CAD build for the part. Positions are in the model's coordinates, mm. Give positions to 0.01 mm unless a question says otherwise; leave off trailing zeros. Write each loop counter-clockwise with the first axis right and the second up, starting at its lowest first coordinate (ties: lowest second). Pieces come first, ordered by that corner, then holes. Notation, with made-up numbers: (-33.5, 24.25) - (-4.5, 24.25) arc R16 cw to (-4.5, 55.25) - close; hole circle Ø6 at (-1, 80.25). An arc over 180 degrees is marked (long way). Put each result on its own line as item: value. Start each with the question number.
1. Wall check: line 1 (Z direction, x = -77.5, y = 4); line 2 (Z direction, x = -127.3, y = 2.5); line 3 (X direction, y = 3, z = 112.3). Give the ranges that are in metal, low to high.
2. Drop a flat-ended pin along its axis: pin 1 (4 mm diameter, centred on x = 105.5, z = -42.5, fed in from -Y). Give the stop position or say it passes through.
3. Cut at A-A on x = -93.45. List the corners of the cut face in (y, z).
4. Cut at B-B on z = 0. List the corners of the cut face in (x, y), and give its area (3 significant figures).
from build123d import *

# Parameters (mm, degrees)
SKETCH1_W               = 280
SKETCH1_H               = 250
BOSS_EXTRUDE1_DEPTH     = 6.35
SKETCH3_R               = 2.38125
CUT_EXTRUDE1_DEPTH      = 7.35
MIRROR2_COPY_1_SKETCH_R = 2.38125
MIRROR2_COPY_1_DEPTH    = 7.35
SKETCH7_R               = 1.55
SKETCH7_R_2             = 11.5
CUT_EXTRUDE4_DEPTH      = 7.35


with BuildPart() as part:
    # Sketch1 → Boss-Extrude1 (new body)
    with BuildSketch(Plane(origin=(0, 0, 0), x_dir=(1, 0, 0), z_dir=(0, 1, 0))):
        Rectangle(SKETCH1_W, SKETCH1_H)
    extrude(amount=BOSS_EXTRUDE1_DEPTH)

    # Sketch3 → Cut-Extrude1 (cut, through all)
    with BuildSketch(Plane(origin=(0, 6.35, 0), x_dir=(1, 0, 0), z_dir=(0, 1, 0))):
        with Locations((-127.3, -112.3)):
            Circle(SKETCH3_R)
    cut_extrude1 = extrude(amount=-CUT_EXTRUDE1_DEPTH, mode=Mode.SUBTRACT)

    # Mirror1: Cut-Extrude1 across plane
    add(cut_extrude1.mirror(Plane.XY), mode=Mode.SUBTRACT)

    # Mirror2: Cut-Extrude1 across plane
    add(cut_extrude1.mirror(Plane(origin=(0, 0, 0), x_dir=(0, 0, 1), z_dir=(1, 0, 0))), mode=Mode.SUBTRACT)

    # Mirror2 copy 1 sketch → Mirror2 copy 1 (cut, through all)
    with BuildSketch(Plane(origin=(0, 6.35, 0), x_dir=(-1, 0, 0), z_dir=(0, 1, 0))):
        with Locations((-127.3, -112.3)):
            Circle(MIRROR2_COPY_1_SKETCH_R)
    extrude(amount=-MIRROR2_COPY_1_DEPTH, mode=Mode.SUBTRACT)

    # Sketch7 → Cut-Extrude4 (cut, through all)
    with BuildSketch(Plane(origin=(0, 6.35, 0), x_dir=(-1, 0, 0), z_dir=(0, 1, 0))):
        with Locations((77.95, 15.5)):
            Circle(SKETCH7_R)
        with Locations((93.45, 0)):
            Circle(SKETCH7_R_2)
        with Locations((108.95, 15.5)):
            Circle(SKETCH7_R)
        with Locations((108.95, -15.5)):
            Circle(SKETCH7_R)
        with Locations((77.95, -15.5)):
            Circle(SKETCH7_R)
    extrude(amount=-CUT_EXTRUDE4_DEPTH, mode=Mode.SUBTRACT)


solid = part.part
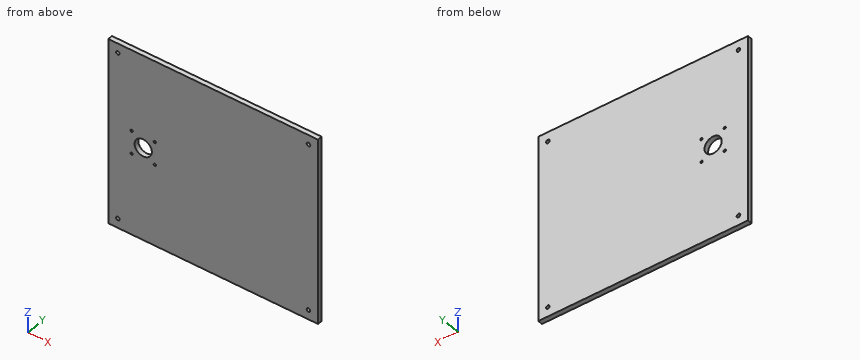
Report:
1. line 1: z = -125 to -16.98, -14.02 to 14.02, 16.98 to 125
1. line 2: z = -125 to -114.68, -109.92 to 109.92, 114.68 to 125
1. line 3: x = -140 to -129.68, -124.92 to 124.92, 129.68 to 140
2. pin 1: stops at y = 0
3. outline: (0, -125) - (6.35, -125) - (6.35, -11.5) - (0, -11.5) - close; (0, 11.5) - (6.35, 11.5) - (6.35, 125) - (0, 125) - close
4. outline: (-140, 0) - (-104.95, 0) - (-104.95, 6.35) - (-140, 6.35) - close; (-81.95, 0) - (140, 0) - (140, 6.35) - (-81.95, 6.35) - close
4. area: 1,630 mm²
